Design review of the part built by this model. Coordinates are the model's own, in mm. A direction names the side the tool comes from. Give positions to 0.01 mm unless a question says otherwise; leave off trailing zeros. Order: outer loops, then holes, each group sorted by start corner. A loop starts at its lowest first (then second) coordinate and runs counter-clockwise, first axis right, second up. Notation, with made-up numbers: (80, 6.5) -> (137, 6.5) arc R24 ccw to (137, 26.5) -> close; hole circle Ø2 at (16, 83). An arc over 180 degrees is marked (long way). One line per item, written item: value.
Autodesk Inventor part; units mm, degrees
ref_plane "YZ Plane" through (0, 0, 0) normal (1, 0, 0) x (0, 1, 0)
ref_plane "XZ Plane" through (0, 0, 0) normal (0, 1, 0) x (-1, 0, 0)
ref_plane "XY Plane" through (0, 0, 0) normal (0, 0, 1) x (1, 0, 0)
sketch "Skizze1" plane through (0, 0, 0) normal (0, 0, 1) x (1, 0, 0)
  circle A0 centre (0, 0) radius 33.35 construction
  circle A1 centre (0, 0) radius 34.95
  circle A2 centre (0, 0) radius 3.6
  circle A3 centre (0, 0) radius 5.6
  circle A4 centre (0, 0) radius 33.45
  circle A5 centre (0, 0) radius 2.6
  line L0 (0, 51.4164) -> (0, -49.3444) construction
  line L1 (-54.4561, 0) -> (54.4561, 0) construction
  line L2 (-2, 30.284) -> (-2, 7.3321)
  line L3 (0, 0) -> (-28.9685, 16.725) construction
  line L4 (-27.2267, -13.41) -> (-7.3498, -1.934)
  arc A6 (-2, 7.3321) -> (-7.3498, -1.934) centre (0, 0) ccw
  arc A7 (-2, 30.284) -> (-27.2267, -13.41) centre (0, 0) ccw
  line L5 (25.2267, -16.8741) -> (5.3498, -5.3981)
  arc A8 (-25.2267, -16.8741) -> (25.2267, -16.8741) centre (0, 0) ccw
  line L6 (-25.2267, -16.8741) -> (-5.3498, -5.3981)
  arc A9 (-5.3498, -5.3981) -> (5.3498, -5.3981) centre (0, 0) ccw
  line L7 (2, 30.284) -> (2, 7.3321)
  arc A10 (27.2267, -13.41) -> (2, 30.284) centre (0, 0) ccw
  line L8 (27.2267, -13.41) -> (7.3498, -1.934)
  arc A11 (7.3498, -1.934) -> (2, 7.3321) centre (0, 0) ccw
  circle A12 centre (0, 0) radius 32.35
  dimension "d1" = 33.35
  dimension "d2" = 7.2
  dimension "d3" = 2
  dimension "d4" = 0.1
  dimension "d5" = 1.5
  dimension "d12" = 1
  dimension "d17" = 60
  dimension "d18" = 2
  dimension "d19" = 3
  dimension "d20" = 2
  dimension "d23" = 360
  dimension "d25" = 1
extrude "Extrusion1" add sketch "Skizze1" along normal blind 1.5 contours A1 | A3 | A4 | A12
extrude "Extrusion2" add sketch "Skizze1" along normal blind 7 from surface at 1.5 contours A1
extrude "Extrusion3" add sketch "Skizze1" against normal blind 3 from surface at 0 contours A3
extrude "Extrusion4" add sketch "Skizze1" against normal blind 1.5 from surface at -3 contours A2 | A3
extrude "Extrusion5" add sketch "Skizze1" along normal blind 4 from surface at 1.5 contours A4
properties part number "ShaftHolder"
Item 1: Add section D-D on z = 4. Give the boundary of the cut face in (x, y), plus the area to 3 significant figures.
Returned:
outline: circle Ø69.9 at (0, 0); hole circle Ø64.7 at (0, 0)
area: 550 mm²
Item 2: To check wall thickness, follow line 1 along Y through (x, z) = (0, 0.25); line 2 along Y through (x, z) = (0, -0.5); line 3 along Y through (x, z) = (0, 3.6). State the ranges of each line that lie inside material, in increasing order. Write a range as from..to.
Returned:
line 1: -34.95..-30.35, -7.6..-3.6, 3.6..34.95
line 2: -5.6..-3.6, 3.6..5.6
line 3: -34.95..-32.35, 32.35..34.95
Item 3: Clearance check with flat-ended pins moving along their axes: P1, Ø1.5, axis at x = -19.5, y = 24.5, coming from the -Z side; P2, Ø3, axis at y = 10, z = 6.5, coming from the -X side; P3, Ø1.6, axis at y = 13.5, z = 0.5, coming from the +X side. State where each tip first meets the part, or that it passes through.
Returned:
P1: z = 0
P2: x = -33.9
P3: x = 32.56
Item 4: Draft analysis for pull direction Y (two halves, no side actions). For faces 1 (the cylindrical face through (3.434, -1.081, -0.781)), 2 (the flat face through (-5, -5, 0)), 3 (the cylindrical face through (-25.76, -23.62, 4.19)), state which applies: pulls with the +Y half, pulls with the -Y half, needs draft (parallel to the pull), parting line crosses it, or undercut.
Returned:
face 1: undercut
face 2: needs draft
face 3: parting line crosses it
Item 5: Add section A-A on y = 0. Count the separate pieces of the cut face and the enclosed holes in it, plus the area to 3 significant figures.
Returned:
separate pieces: 4
enclosed holes: 0
area: 76.6 mm²
Item 6: Machinability: for faces 4 (the flat face through (-17.5, 27.4, 5.5)), 5 (the flat face through (-3, -1, -4.5)), 6 (the flat face through (-2, 19, 1)), 7 (the cylindrical face through (-5.595, 0.246, -2.218)), which of the approach directions +Z, -Z, +X, -X, +Y, -Y give a long, thin tool a straight path to every point of the face, cutting with its end or side? Answer none if there is none.
Returned:
face 4: +Z
face 5: -Z, +X, -X, +Y, -Y
face 6: +Z, -Z
face 7: -Z
Item 7: Add section B-B on x = 0. Give the boundary of the cut face in (y, z), plus the area to 3 significant figures.
Returned:
outline: (-34.95, 0) -> (-30.35, 0) -> (-30.35, 1.5) -> (-32.35, 1.5) -> (-32.35, 5.5) -> (-33.45, 5.5) -> (-33.45, 8.5) -> (-34.95, 8.5) -> close; (-7.6, 0) -> (-5.6, 0) -> (-5.6, -4.5) -> (-2.6, -4.5) -> (-2.6, -3) -> (-3.6, -3) -> (-3.6, 1.5) -> (-7.6, 1.5) -> close; (2.6, -4.5) -> (5.6, -4.5) -> (5.6, 0) -> (34.95, 0) -> (34.95, 8.5) -> (33.45, 8.5) -> (33.45, 5.5) -> (32.35, 5.5) -> (32.35, 1.5) -> (3.6, 1.5) -> (3.6, -3) -> (2.6, -3) -> close
area: 111 mm²
Item 8: Add section C-C on y = 14.5. Give the boundary of the cut face in (x, z).
Returned:
outline: (-31.8, 0) -> (-26.66, 0) -> (-26.66, 1.5) -> (-28.92, 1.5) -> (-28.92, 5.5) -> (-30.14, 5.5) -> (-30.14, 8.5) -> (-31.8, 8.5) -> close; (-2, 0) -> (2, 0) -> (2, 1.5) -> (-2, 1.5) -> close; (26.66, 0) -> (31.8, 0) -> (31.8, 8.5) -> (30.14, 8.5) -> (30.14, 5.5) -> (28.92, 5.5) -> (28.92, 1.5) -> (26.66, 1.5) -> close
